Read the model definition and answer for the solid it produces. Units are mm, in the model's axes. Face numbers are marked on the shaded views. A direction names the side the tool comes from. Coordinates: 2 decimals unless noted, no trailing zeros. Order: outer loops, then holes, each group sorted by start corner. A loop starts at its lowest first (then second) coordinate and runs counter-clockwise, first axis right, second up.
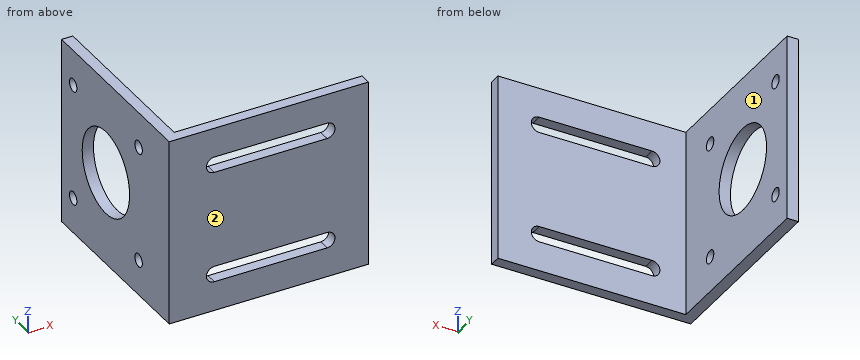
```python
from build123d import *

# Parameters (mm, degrees)
EXTRUDE_1_DEPTH     = 50
SKETCH_3_R          = 11.223257521
SKETCH_3_R_2        = 1.75
CUT_EXTRUDE_1_DEPTH = 76.168144849
CUT_EXTRUDE_2_DEPTH = 75.204110398


with BuildPart() as part:
    # 草图2 → 凸台-拉伸1 (new body)
    with BuildSketch(Plane.XY):
        Polygon((-23.5, 25.5), (-23.5, -22.5), (26.5, -22.5), (26.5, -25.5), (-26.5, -25.5), (-26.5, 25.5), align=None)
    extrude(amount=EXTRUDE_1_DEPTH)

    # 草图3 → 切除-拉伸1 (cut, through all)
    with BuildSketch(Plane(origin=(-23.5, 0, 0), x_dir=(0, 0, -1), z_dir=(1, 0, 0))):
        with Locations(Location((-25, 4.5, 0), (0, 0, 90))):
            Circle(SKETCH_3_R)
        with Locations(Location((-40.5, 20, 0), (0, 0, 90))):
            Circle(SKETCH_3_R_2)
        with Locations(Location((-9.5, 20, 0), (0, 0, 90))):
            Circle(SKETCH_3_R_2)
        with Locations(Location((-9.5, -11, 0), (0, 0, 90))):
            Circle(SKETCH_3_R_2)
        with Locations(Location((-40.5, -11, 0), (0, 0, 90))):
            Circle(SKETCH_3_R_2)
    extrude(amount=-CUT_EXTRUDE_1_DEPTH, mode=Mode.SUBTRACT)

    # 草图4 → 切除-拉伸2 (cut, through all)
    with BuildSketch(Plane(origin=(0, -22.5, 0), x_dir=(1, 0, 0), z_dir=(0, 1, 0))):
        with BuildLine():
            Line((-14.5, -7.9), (15.5, -7.9))
            ThreePointArc((15.5, -7.9), (17.6, -10), (15.5, -12.1))
            Line((15.5, -12.1), (-14.5, -12.1))
            ThreePointArc((-14.5, -12.1), (-16.6, -10), (-14.5, -7.9))
        make_face()
        with BuildLine():
            Line((15.5, -37.9), (-14.5, -37.9))
            ThreePointArc((-14.5, -37.9), (-16.6, -40), (-14.5, -42.1))
            Line((-14.5, -42.1), (15.5, -42.1))
            ThreePointArc((15.5, -42.1), (17.6, -40), (15.5, -37.9))
        make_face()
    extrude(amount=-CUT_EXTRUDE_2_DEPTH, mode=Mode.SUBTRACT)


solid = part.part
```
1) A cutting plane is placed at A-A, the plane y = -11. Determine the outline of the cut face in (x, z).
A:
outline: (-26.5, 0) - (-23.5, 0) - (-23.5, 7.75) - (-26.5, 7.75) - close; (-26.5, 11.25) - (-23.5, 11.25) - (-23.5, 38.75) - (-26.5, 38.75) - close; (-26.5, 42.25) - (-23.5, 42.25) - (-23.5, 50) - (-26.5, 50) - close
2) A cutting plane is placed at C-C, the plane y = 8.5. Determine the outline of the cut face in (x, z), and give its area (3 significant figures).
A:
outline: (-26.5, 0) - (-23.5, 0) - (-23.5, 14.51) - (-26.5, 14.51) - close; (-26.5, 35.49) - (-23.5, 35.49) - (-23.5, 50) - (-26.5, 50) - close
area: 87.1 mm2
3) Which of the six approach directions +Z, -Z, +X, -X, +Y, -Y give full straight-line access (tool end or side, diameter ignored) to the marked faces 1 and 2?
A:
face 1: +Z, -Z, +X, +Y
face 2: +Z, -Z, +X, -X, -Y
4) A cutting plane is placed at D-D, the plane z = 3.5. Determine the outline of the cut face in (x, y), and give its area (3 significant figures).
A:
outline: (-26.5, -25.5) - (26.5, -25.5) - (26.5, -22.5) - (-23.5, -22.5) - (-23.5, 25.5) - (-26.5, 25.5) - close
area: 303 mm2
5) A cutting plane is placed at B-B, the plane z = 25. Determine the outline of the cut face in (x, y).
A:
outline: (-26.5, -25.5) - (26.5, -25.5) - (26.5, -22.5) - (-23.5, -22.5) - (-23.5, -6.72) - (-26.5, -6.72) - close; (-26.5, 15.72) - (-23.5, 15.72) - (-23.5, 25.5) - (-26.5, 25.5) - close
6) Flat-ended cylindrical pins translate along their axes: pin 1 Ø2 at (y, z) = (-11, 40.5) entering from +X; pin 2 Ø1.5 at (y, z) = (3.5, 45) entering from +X; pin 3 Ø10 at (x, z) = (5, 9) entering from +Y. Find the tip coordinate at first contact, or state that the pin passes through.
A:
pin 1: passes through
pin 2: stops at x = -23.5
pin 3: stops at y = -22.5
7) Straight lines are drawn through the part: line 1 (Z direction, x = -25.25, y = 20); line 2 (X direction, y = -16.5, z = 11); line 3 (Y direction, x = 17, z = 16.5). For each, find the intervals that lie inside material, in ascending order.
A:
line 1: z = 0 to 7.75, 11.25 to 38.75, 42.25 to 50
line 2: x = -26.5 to -23.5
line 3: y = -25.5 to -22.5
